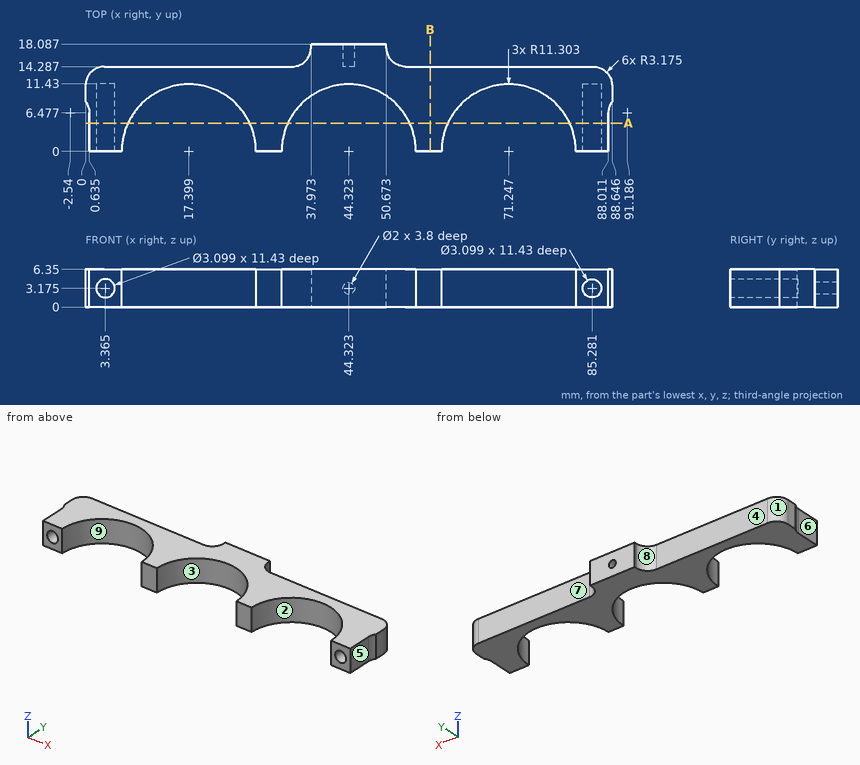
Job drawing, mm, ordinate dimensions from the low corner. One solid piece. A direction names the side the tool comes from. Give positions to 0.01 mm unless a question says otherwise; leave off trailing zeros. Write each loop counter-clockwise with the first axis right and the second up, starting at its lowest first coordinate (ties: lowest second). Pieces come first, ordered by that corner, then holes. Notation, with made-up numbers: M 42,-18.75 L 73,-18.75 A20 ccw 73,-6.75 Z; hole C -30,12 d9. An arc over 180 degrees is marked long. Put each result on its own line as item: value. Start each with the question number.
(1) Which spindle directions (+Z, -Z, +X, -X, +Y, -Y) get a long thin tool onto all of the face, cutting with end or side? Do the marked faces 5, 6, 7, 8 and 9. Say none if no direction does.
(2) Band-saw the part on B-B, the plane x = 58. Write the cut outline in (y, z).
(3) Mould opens along X. For the marked faces 1, 2, 3 and 4 say: +X half, -X half, draft (parallel to the pull), parting line (faces both ways), or undercut.
(4) Flat gauge pins, fed straight in: pin 1 Ø1.6 at (x, z) = (44.5, 3.5) entering from +Y; pin 2 Ø0.5 at (y, z) = (18, 2.5) entering from -X; pin 3 Ø1.8 at (x, z) = (44.323, 3.175) entering from +Y; pin 4 Ø1.5 at (x, z) = (85, 3.5) entering from -Y. Where does each tip first touch, or does it go through?
(5) Probe L1, parallel to Y at x = 25, z = 1.5 (1 decimal); L2, parallel to Y at x = 5, z = 5; L3, parallel to X at y = 16.25, z = 1 (1 decimal). List the from-to ranges inside material, lowest first.
(6) Band-saw the part on A-A, the plane y = 4.75. Give the number of separate pieces and of enclosed holes in the cut face, and give its area (3 significant figures).
Response values:
1. face 5: +Z, -Z, +X, -Y
1. face 6: +Z, -Z, -X, -Y
1. face 7: +Z, -Z, +X, +Y
1. face 8: +Z, -Z, -X, +Y
1. face 9: +Z, -Z, -Y
2. outline: M 0,0 L 14.29,0 L 14.29,6.35 L 0,6.35 Z
3. face 1: -X half
3. face 2: undercut
3. face 3: undercut
3. face 4: draft
4. pin 1: stops at y = 18.09
4. pin 2: stops at x = 37.97
4. pin 3: stops at y = 14.29
4. pin 4: stops at y = 11.43
5. L1: y = 8.4 to 14.3
5. L2: y = 0 to 14.29
5. L3: x = 37.7 to 50.9
6. separate pieces: 4
6. enclosed holes: 2
6. area: 149 mm2
